Job drawing, mm, ordinate dimensions from the low corner. One solid piece. A direction names the side the tool comes from. Give positions to 0.01 mm unless a question says otherwise; leave off trailing zeros. Order: outer loops, then holes, each group sorted by start corner. A loop starts at its lowest first (then second) coordinate and runs counter-clockwise, first axis right, second up. Notation, with made-up numbers: (-36.75, -38) - (-22.75, -38) arc R20 cw to (-22.75, -11) - close; hole circle Ø11 at (64.25, 17.5). An arc over 180 degrees is marked (long way). One line per item, written item: value.
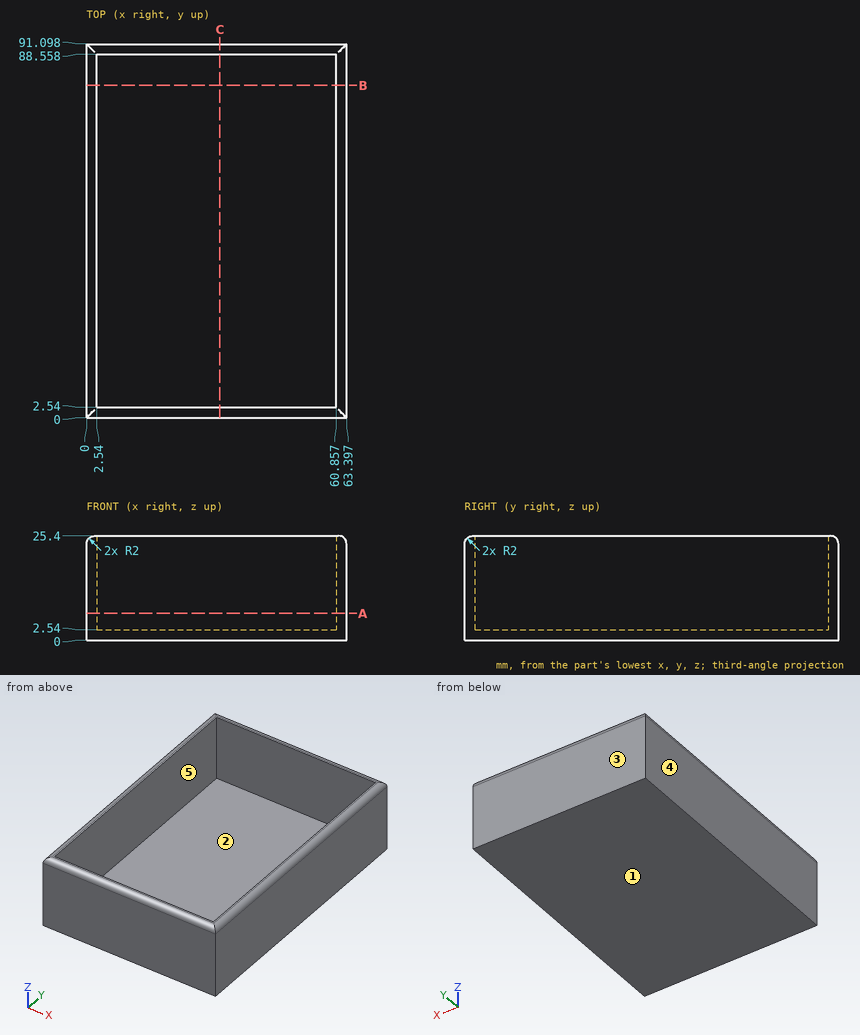
1) Drop a flat-ended pin along its axis: P1, Ø17.5, axis at x = 36, y = 41, coming from the +Z side. Give the stop position or say it passes through.
Answer:
P1: stops at z = 2.54
2) Slice it at A-A on z = 6.5. Write the cut outline in (x, y), then the cut area to 3 significant figures.
Answer:
outline: (0, 0) - (63.4, 0) - (63.4, 91.1) - (0, 91.1) - close; hole (2.54, 2.54) - (60.86, 2.54) - (60.86, 88.56) - (2.54, 88.56) - close
area: 759 mm2
3) Two-plate mould, pull along Y, no slides. Class the marked faces 1, 2 and 3: pulls with the +Y half, pulls with the -Y half, needs draft (parallel to the pull), parting line crosses it, or undercut.
Answer:
face 1: needs draft
face 2: undercut
face 3: pulls with the +Y half
4) Wall check: line 1 along Y through (x, z) = (3.5, 19.25); line 2 along X through (y, z) = (38, 7.25); line 3 along Z through (x, y) = (22, 8). Give the ranges that are in metal, low to high. Write a range as [from, to].
Answer:
line 1: y = [0, 2.54], [88.56, 91.1]
line 2: x = [0, 2.54], [60.86, 63.4]
line 3: z = [0, 2.54]
5) Slice it at C-C on x = 32.5. Write the cut outline in (y, z), then the cut area to 3 significant figures.
Answer:
outline: (0, 0) - (91.1, 0) - (91.1, 23.4) arc R2 ccw to (89.1, 25.4) - (88.56, 25.4) - (88.56, 2.54) - (2.54, 2.54) - (2.54, 25.4) - (2, 25.4) arc R2 ccw to (0, 23.4) - close
area: 346 mm2
6) Which spindle directions (+Z, -Z, +X, -X, +Y, -Y) get a long thin tool onto all of the face, cutting with end or side? Do the marked faces 4 and 5. Say none if no direction does.
Answer:
face 4: +Z, -Z, -X, +Y, -Y
face 5: +Z
7) Slice it at B-B on y = 81. Write the cut outline in (x, z).
Answer:
outline: (0, 0) - (63.4, 0) - (63.4, 23.4) arc R2 ccw to (61.4, 25.4) - (60.86, 25.4) - (60.86, 2.54) - (2.54, 2.54) - (2.54, 25.4) - (2, 25.4) arc R2 ccw to (0, 23.4) - close
